Autodesk Inventor part; units mm, degrees
ref_plane "YZ Plane" through (0, 0, 0) normal (1, 0, 0) x (0, 1, 0)
ref_plane "XZ Plane" through (0, 0, 0) normal (0, 1, 0) x (-1, 0, 0)
ref_plane "XY Plane" through (0, 0, 0) normal (0, 0, 1) x (1, 0, 0)
sketch "Sketch1" plane through (0, 0, 0) normal (0, 0, 1) x (1, 0, 0)
  line L0 (-18.7296, 9.1612) -> (16.5704, 9.1612)
  line L1 (16.5704, 9.1612) -> (16.5704, -0.3388)
  line L2 (16.5704, -0.3388) -> (-18.7296, -0.3388)
  line L3 (-18.7296, -0.3388) -> (-18.7296, 9.1612)
  line L4 (-18.7296, 4.4112) -> (16.5704, 4.4112)
  line L5 (-18.7296, 4.4112) -> (-18.7296, -0.3388)
  line L6 (-18.7296, 2.0362) -> (16.5704, 2.0362)
  line L7 (16.5704, 4.4112) -> (14.1954, 2.0362)
  line L8 (16.5704, 4.4112) -> (19.9291, 4.4112) construction
  line L9 (-18.7296, 4.4112) -> (-16.3546, 2.0362)
  line L10 (-16.3546, 2.0362) -> (-16.3546, 9.1612)
  line L11 (14.1954, 2.0362) -> (14.1954, 9.1612)
  line L12 (-16.3546, 4.4112) -> (-13.9796, 2.0362)
  line L13 (14.1954, 4.4112) -> (11.8204, 2.0362)
  line L14 (11.8204, 2.0362) -> (11.8204, 9.1612)
  line L15 (-13.9796, 2.0362) -> (-13.9796, 9.1612)
  point P0 (0, 0)
  dimension "d0" = 35.3
  dimension "d1" = 9.5
  dimension "d2" = 135
extrude "Extrusion1" add sketch "Sketch1" along normal blind 445 contours L0 L15 L4 L10 | L12 L6 L10 | L4 L15 L12 | L0 L11 L4 L14 | L4 L14 L6 L15 | L4 L13 L14 | L13 L11 L6
sketch "Sketch2" plane through (-13.9796, 4.4112, 0) normal (0, 1, 0) x (1, 0, 0)
  line L0 (0, -445) -> (25.8, -445)
  line L1 (12.9, -445) -> (12.9, -416.7)
  circle A0 centre (12.9, -416.7) radius 2.15
  line L2 (12.9, -416.7) -> (12.9, -64.7)
  circle A1 centre (12.9, -64.7) radius 2.15
  line L3 (12.9, -416.7) -> (12.9, -32.7)
  circle A2 centre (12.9, -32.7) radius 2.15
  point P0 (13.9796, 0)
  dimension "d5" = 28.3
  dimension "d6" = 4.3
  dimension "d7" = 352
  dimension "d8" = 384
extrude "Extrusion2" cut sketch "Sketch2" against normal blind 445
sketch "Sketch3" plane through (0, 0, 445) normal (0, 0, 1) x (1, 0, 0)
  line L0 (14.1954, 2.0362) -> (-16.3546, 2.0362)
  line L1 (14.1954, 9.1612) -> (14.1954, 2.0362)
  line L2 (11.8204, 9.1612) -> (14.1954, 9.1612)
  line L3 (11.8204, 4.4112) -> (11.8204, 9.1612)
  line L4 (-13.9796, 4.4112) -> (11.8204, 4.4112)
  line L5 (-13.9796, 9.1612) -> (-13.9796, 4.4112)
  line L6 (-16.3546, 9.1612) -> (-13.9796, 9.1612)
  line L7 (-16.3546, 2.0362) -> (-16.3546, 9.1612)
  point P0 (0, 0)
extrude "Extrusion3" cut sketch "Sketch3" against normal blind 419.1
sketch "Sketch4" plane through (0, 0, 0) normal (0, 0, -1) x (-1, 0, 0)
  line L0 (-14.1954, 2.0362) -> (-14.1954, 9.1612)
  line L1 (16.3546, 2.0362) -> (-14.1954, 2.0362)
  line L2 (16.3546, 9.1612) -> (16.3546, 2.0362)
  line L3 (13.9796, 9.1612) -> (16.3546, 9.1612)
  line L4 (13.9796, 4.4112) -> (13.9796, 9.1612)
  line L5 (-11.8204, 4.4112) -> (13.9796, 4.4112)
  line L6 (-11.8204, 9.1612) -> (-11.8204, 4.4112)
  line L7 (-14.1954, 9.1612) -> (-11.8204, 9.1612)
  point P0 (0, 0)
extrude "Extrusion4" add sketch "Sketch4" against normal blind 422.275
sketch "Sketch5" plane through (-16.3546, 2.0362, 0) normal (0, -1, 0) x (1, 0, 0)
  line L0 (30.55, 422.275) -> (0, 422.275)
  line L1 (15.275, 422.275) -> (15.275, 331.216)
  circle A0 centre (15.275, 331.216) radius 2.3495
  line L2 (15.275, 422.275) -> (15.275, 187.325)
  circle A1 centre (15.275, 187.325) radius 2.3495
  point P0 (16.3546, 0)
  dimension "d15" = 91.059
  dimension "d16" = 4.699
  dimension "d17" = 234.95
extrude "Extrusion5" cut sketch "Sketch5" against normal blind 422.275
sketch "Sketch6" plane through (-16.3546, 2.0362, 0) normal (0, -1, 0) x (1, 0, 0)
  line L0 (30.55, 422.275) -> (0, 422.275)
  line L1 (15.275, 422.275) -> (15.275, 417.83)
  circle A0 centre (15.275, 417.83) radius 2.3495
  point P0 (16.3546, 0)
  dimension "d20" = 4.445
extrude "Extrusion6" cut sketch "Sketch6" against normal blind 422.275
properties part number "2"
The listing builds one solid part. Answer for the finished solid, in the listing's coordinates (mm). Round coordinates to 2 decimals unless told otherwise and drop trailing zeros. Write each loop counter-clockwise with the first axis right and the second up, starting at its lowest first coordinate (ties: lowest second). Pieces come first, ordered by that corner, then holes. Notation, with made-up numbers: (-38, 54.5) -> (8, 54.5) arc R29 ccw to (8, 90.5) -> close; hole circle Ø9 at (88, 40). An arc over 180 degrees is marked (long way). Answer as a JSON object with one key per item and string values. Group by question number.
Q1. Straight lines are drawn through the part: line 1 along X through (y, z) = (7.5, 44); line 2 along Z through (x, y) = (-2, 4) (3 decimals); line 3 along X through (y, z) = (3.15, 417.83). For each, find the intervals that lie inside material, in ascending order.
Q2. This flat-tipped pin is pushed along its axis until it touches: pin 1 Ø8 at (x, z) = (7.5, 145) entering from +Y. Where does it stop, or does it pass through?
Q3. Determine the mould class of faces 1 (the face through (-1, 2.036, 208)), 2 (the face through (14.195, 6, 208)), 3 (the face through (-1, 4.411, 208)) for opening direction X: pulls with the +X half, pulls with the -X half, needs draft (parallel to the pull), parting line crosses it, or undercut.
Q4. Section B-B (z = 167.5) is taken. Write down the section's boundary in (x, y), plus the area to 3 significant figures.
Q5. Section A-A (y = 5.5) is taken. Write down the section's boundary in (x, z) (3 decimals).
Check values:
{
 "1": {"line 1": "-16.35 to -13.98, 11.82 to 14.2", "line 2": "0 to 185.163, 189.487 to 329.054, 333.378 to 415.668, 419.992 to 422.275", "line 3": "-16.35 to -3.43, 1.27 to 14.2"},
 "2": {"pin 1": "y = 4.41"},
 "3": {"face 1": "needs draft", "face 2": "pulls with the +X half", "face 3": "undercut"},
 "4": {"outline": "(-16.35, 2.04) -> (14.2, 2.04) -> (14.2, 9.16) -> (11.82, 9.16) -> (11.82, 4.41) -> (-13.98, 4.41) -> (-13.98, 9.16) -> (-16.35, 9.16) -> close", "area": "95.1 mm^2"},
 "5": {"outline": "(-16.355, 0) -> (-13.98, 0) -> (-13.98, 422.275) -> (-16.355, 422.275) -> close; (11.82, 0) -> (14.195, 0) -> (14.195, 422.275) -> (11.82, 422.275) -> close"}
}
